Can you work these out from the model? Positions are in its coordinate system, mm. Give positions to 0.01 mm unless a question says otherwise; leave off trailing zeros. Loops run counter-clockwise (first coordinate to the right, second up) from the corner with the lowest first, then second, coordinate; pieces in that order, holes last. Notation, with made-up numbers: (41, 66.25) -> (70, 66.25) arc R11 cw to (70, 70.25) -> close; hole circle Ø4 at (47.25, -12.5). An arc over 180 degrees is marked (long way). One line per question, with ' | ' between items.
from build123d import *

# Parameters (mm, degrees)
F2_R = 0.99999
F3_R = 2


# Not quite as in the source:
# - a fillet or chamfer is up to 0.001 mm smaller than in the source, because OpenCascade refuses the exact size


with BuildPart() as f1:
    # F0 (on Front) → F1 (revolve)
    with BuildSketch(Plane.XZ):
        with BuildLine():
            Line((-10.5, 0), (-10.5, 30))
            Line((-10.5, 30), (-13.532049904, 29.9838036175))
            ThreePointArc((-13.532049904, 29.9838036175), (-17.7539569476, 28.2151833802), (-19.5, 23.9838892179))
            Line((-19.5, 23.9838892179), (-19.5, 20))
            Line((-19.5, 20), (-19.5, -20))
            Line((-19.5, -20), (-17.5, -20))
            Line((-17.5, -20), (-17.5, 20))
            Line((-17.5, 20), (-15.5, 20))
            Line((-15.5, 20), (-15.5, 0))
            Line((-15.5, 0), (-10.5, 0))
        make_face()
    revolve(axis=Axis((0, 0, 11.9062974118), (0, 0, -1)))

    # F2 (radius 1 in the source; OpenCascade refuses exactly that, so slightly less here)
    f2_edges = [f1.edges().sort_by_distance(p)[0] for p in [
        (17.5, 0, -20),
        (19.5, 0, -20),
    ]]
    fillet(f2_edges, radius=F2_R)

    # F3
    f3_edges = [f1.edges().sort_by_distance(p)[0] for p in [
        (10.5, 0, 0),
        (15.5, 0, 0),
    ]]
    fillet(f3_edges, radius=F3_R)


solid = f1.part
Q1. If we section it at C-C (z = 17): Write out the boundary of the cut face in (x, y), plus the area to 3 significant figures.
Entries:
outline: circle Ø39 at (0, 0); circle Ø31 at (0, 0); hole circle Ø35 at (0, 0); hole circle Ø21 at (0, 0) | area: 641 mm²
Q2. If we mould it in two halves opening along X, with no side actions, what happens to faces 1 (the face through (2.018, 15.368, 10.874)), 2 (the face through (2.539, 19.334, 2.191))? For each: pulls with the +X half, pulls with the -X half, needs draft (parallel to the pull), parting line crosses it, or undercut.
Entries:
face 1: undercut | face 2: parting line crosses it
Q3. If I drill on probe 1 along Y at (x, z) = (0, 10.5); probe 2 along Y at (x, z) = (1.5, 7); probe 3 along X at (y, z) = (-11.5, 3), over which ranges is the centre line in solid material (lowest first)? Write a range as from..to.
Entries:
probe 1: -19.5..-17.5, -15.5..-10.5, 10.5..15.5, 17.5..19.5 | probe 2: -19.44..-17.44, -15.43..-10.39, 10.39..15.43, 17.44..19.44 | probe 3: -15.75..-13.19, -10.39..10.39, 13.19..15.75
Q4. For pin 1 Ø4 at (x, z) = (-15, 6) entering from +Y; pin 2 Ø1.5 at (y, z) = (-13, -9.5) entering from +X; pin 3 Ø1 at (x, y) = (8.5, 12.5) entering from +Z, each with a flat end and sliding along its axis, tell me the tip position at first contact or that it passes through.
Entries:
pin 1: y = 14.53 | pin 2: x = 15.17 | pin 3: z = 29.88
Q5. If we section it at D-D (z = -2): Write out the boundary of the cut face in (x, y).
Entries:
outline: circle Ø39 at (0, 0); hole circle Ø35 at (0, 0)
